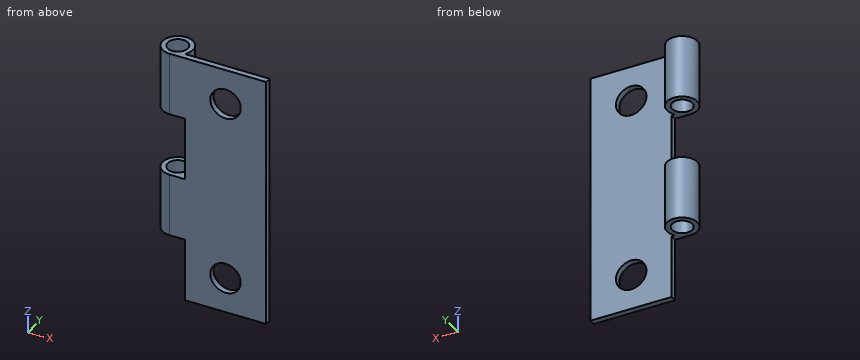
from build123d import *

# Parameters (mm, degrees)
SKETCH_2_R          = 1
EXTRUDE_1_DEPTH     = 12.5
SKETCH_3_W          = 3.539964401
SKETCH_3_H          = 6.25
SKETCH_3_W_2        = 3.996790544
CUT_EXTRUDE_1_DEPTH = 12.5
SKETCH_4_R          = 1.5
CUT_EXTRUDE_2_DEPTH = 10


with BuildPart() as part:
    # 草图2 → 凸台-拉伸1 (new, symmetric)
    with BuildSketch(Plane.XY):
        with BuildLine():
            Line((0, -1.5), (9.5, -1.5))
            Line((9.5, -1.5), (9.5, -0.9))
            Line((9.5, -0.9), (1.2, -0.9))
            ThreePointArc((1.2, -0.9), (-0.670820393, 1.341640786), (0, -1.5))
        make_face()
        Circle(SKETCH_2_R, mode=Mode.SUBTRACT)
    extrude(amount=EXTRUDE_1_DEPTH, both=True)

    # 草图3 → 切除-拉伸1 (cut, symmetric)
    with BuildSketch(Plane(origin=(0, -0.9, 0), x_dir=(1, 0, 0), z_dir=(0, 1, 0))):
        with Locations((-0.238476372, 9.375)):
            Rectangle(SKETCH_3_W, SKETCH_3_H)
        with Locations((-0.466889443, -3.125)):
            Rectangle(SKETCH_3_W_2, SKETCH_3_H)
    extrude(amount=CUT_EXTRUDE_1_DEPTH, both=True, mode=Mode.SUBTRACT)

    # 草图4 → 切除-拉伸2 (cut)
    with BuildSketch(Plane(origin=(0, -0.9, 0), x_dir=(1, 0, 0), z_dir=(0, 1, 0))):
        with Locations(Location((5.5, 9, 0), (0, 0, 180))):
            Circle(SKETCH_4_R)
        with Locations(Location((5.5, -9, 0), (0, 0, 180))):
            Circle(SKETCH_4_R)
    extrude(amount=-CUT_EXTRUDE_2_DEPTH, mode=Mode.SUBTRACT)


solid = part.part
Design review of the part built by this model. Coordinates are the model's own, in mm. Give positions to 0.01 mm unless a question says otherwise; leave off trailing zeros. Loops run counter-clockwise (first coordinate to the right, second up) from the corner with the lowest first, then second, coordinate; pieces in that order, holes last. Notation, with made-up numbers: M -6,66 L 18,66 A28 cw 18,100 Z; hole C 79,31.25 d3. An arc over 180 degrees is marked long. One line per question, with ' | ' between items. Start each with the question number.
1. Insertion check: P1, Ø2.5, axis at x = 5, z = -4.5, coming from the +Y side; P2, Ø4, axis at x = 5.5, z = 8.5, coming from the -Y side; P3, Ø1.2, axis at x = 0, y = 0, coming from the -Z side; P4, Ø1.5, axis at x = 0, y = 0.5, coming from the -Z side. Each pin has a flat end and moves straight along its axis. Give the tip position at first contact, or say it passes through.
2. Add section A-A (z = 9). Write out the cut boundary in (x, y), plus the area to 3 significant figures.
3. Add section C-C (z = -9). Write out the cut boundary in (x, y).
4. Add section B-B (x = 5.5). Write out the cut boundary in (y, z), plus the area to 3 significant figures.
5. Add section D-D (y = 0). Write out the cut boundary in (x, z), plus the area to 3 significant figures.
6. To check wall thickness, follow L1, parallel to Z at x = 5.5, y = -1.05; L2, parallel to Y at x = 2.25, z = 3.5; L3, parallel to X at y = 0, z = -2. State the ranges of each line that lie inside material, in increasing order.
Worked out:
1) P1: stops at y = -0.9 | P2: stops at y = -1.5 | P3: passes through | P4: stops at z = -6.25
2) outline: M 0,-1.5 L 4,-1.5 L 4,-0.9 L 1.2,-0.9 A1.5 ccw long Z; M 7,-1.5 L 9.5,-1.5 L 9.5,-0.9 L 7,-0.9 Z; hole C 0,0 d2 | area: 7.32 mm²
3) outline: M 1.53,-1.5 L 4,-1.5 L 4,-0.9 L 1.53,-0.9 Z; M 7,-1.5 L 9.5,-1.5 L 9.5,-0.9 L 7,-0.9 Z
4) outline: M -1.5,-12.5 L -0.9,-12.5 L -0.9,-10.5 L -1.5,-10.5 Z; M -1.5,-7.5 L -0.9,-7.5 L -0.9,7.5 L -1.5,7.5 Z; M -1.5,10.5 L -0.9,10.5 L -0.9,12.5 L -1.5,12.5 Z | area: 11.4 mm²
5) outline: M -1.5,-6.25 L -1,-6.25 L -1,0 L -1.5,0 Z; M -1.5,6.25 L -1,6.25 L -1,12.5 L -1.5,12.5 Z; M 1,-6.25 L 1.5,-6.25 L 1.5,0 L 1,0 Z; M 1,6.25 L 1.5,6.25 L 1.5,12.5 L 1,12.5 Z | area: 12.5 mm²
6) L1: z = -12.5 to -10.5, -7.5 to 7.5, 10.5 to 12.5 | L2: y = -1.5 to -0.9 | L3: x = -1.5 to -1, 1 to 1.5
